Could you check a few things on this drawing? It's one solid part, dimensions in mm from its lowest x, y, z. Give positions to 0.01 mm unless a question says otherwise; leave off trailing zeros. Write each loop counter-clockwise with the first axis right and the second up, starting at its lowest first coordinate (ties: lowest second). Pieces come first, ordered by that corner, then holes. Notation, with made-up numbers: (34.5, 71.5) - (64.5, 71.5) arc R17 ccw to (64.5, 86.5) - close; hole circle Ø9 at (-32.75, 53). An arc over 180 degrees is marked (long way). One line per item, written item: value. Start each with the question number.
1) I'm going to push a flat-ended pin straight in: P1, Ø0.5, axis at y = 13.5, z = 0.5, coming from the +X side. Where does the tip first touch, or does it pass through?
2) Imagine slicing it at B-B on x = 8.75. Write out the boundary of the cut face in (y, z).
3) Please list where these lines run through material, in increasing order: L1, parallel to Y at x = 11.75, z = 0.65; L2, parallel to X at y = 5, z = 0.85. Write a range as [from, to].
4) Imagine slicing it at A-A on z = 0.65. Write out the boundary of the cut face in (x, y).
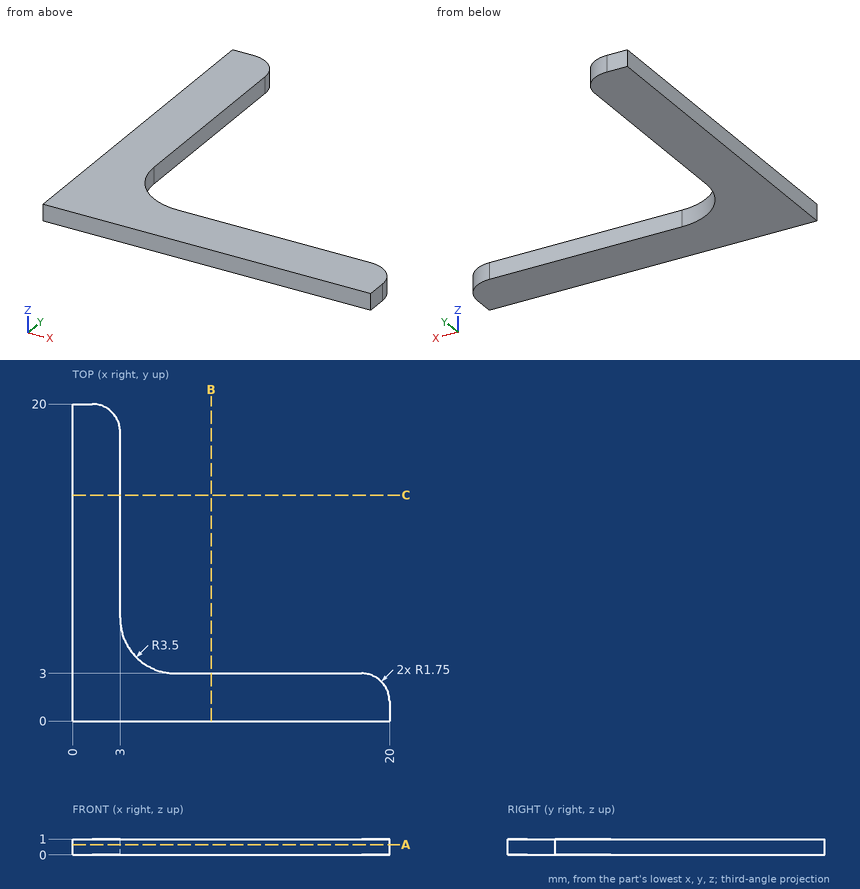
Numbers:
1. P1: x = 3
2. outline: (0, 0) - (3, 0) - (3, 1) - (0, 1) - close
3. L1: [0, 3]
3. L2: [0, 3.34]
4. outline: (0, 0) - (20, 0) - (20, 1.25) arc R1.75 ccw to (18.25, 3) - (6.5, 3) arc R3.5 cw to (3, 6.5) - (3, 18.25) arc R1.75 ccw to (1.25, 20) - (0, 20) - close
